from build123d import *

# Parameters (mm, degrees)
F2_DEPTH = 5.08
F3_R     = 16.9333333333
F4_DEPTH = 5.08
F5_DEPTH = 5.08


# Not quite as in the source:
# - a variable given as a bare number and used for a length is read in inches; the dataset says mm whatever the document's units were


with BuildPart() as f2:
    # F1 (on Top) → F2 (new body)
    with BuildSketch(Plane.XY):
        with BuildLine():
            ThreePointArc((100.8237705737, -47.527355603), (134.6904372404, -13.6606889364), (100.8237705737, 20.2059777303))
            Line((100.8237705737, 20.2059777303), (-102.3762294263, 20.2059777303))
            ThreePointArc((-102.3762294263, 20.2059777303), (-136.2428960929, -13.6606889364), (-102.3762294263, -47.527355603))
            Line((-102.3762294263, -47.527355603), (100.8237705737, -47.527355603))
        make_face()
    extrude(amount=F2_DEPTH)

    # F3 (on face) → F4 (join)
    with BuildSketch(Plane(origin=(0, 0, 0), x_dir=(1, 0, 0), z_dir=(0, 0, -1))):
        with Locations((-102.3762294263, 13.6606889364)):
            Circle(F3_R)
    extrude(amount=F4_DEPTH)

    # F3 (on face) → F5 (cut)
    with BuildSketch(Plane(origin=(0, 0, 0), x_dir=(1, 0, 0), z_dir=(0, 0, -1))):
        with Locations((100.8237705737, 13.6606889364)):
            Circle(F3_R)
    extrude(amount=-F5_DEPTH, mode=Mode.SUBTRACT)


solid = f2.part
For this review, take the finished solid that the model builds, in its own axes (mm). A direction names the side the tool comes from. Coordinates: 2 decimals unless noted, no trailing zeros. Loops run counter-clockwise (first coordinate to the right, second up) from the corner with the lowest first, then second, coordinate; pieces in that order, holes last. Notation, with made-up numbers: (62, -5) - (84, -5) arc R25 ccw to (84, 30) - close; hole circle Ø9 at (-4.75, 81.25). An arc over 180 degrees is marked (long way). Use a Markdown table: item, result. Add a question column.
Item 1: We need section D-D (x = -26). Give the boundary of the cut face in (y, z), and give its area (3 significant figures).
Item 2: For line 1 (Z direction, x = 40, y = 2.5); line 2 (Y direction, x = 97, z = 2); line 3 (X direction, y = -18.5, z = 0.5), list the stretches that pass through material, from the lowest coordinate up.
Item 3: Mouldability with a two-part tool opening along X and no side actions: class faces 1 (the face through (-3, -13, 0)), 2 (the face through (87.386, -3.357, 2.504)), 3 (the face through (-136.235, -12.916, 2.504)) as pulls with the +X half, pulls with the -X half, needs draft (parallel to the pull), parting line crosses it, or undercut.
Item 4: We need section B-B (x = 97). Give the boundary of the cut face in (y, z), and give its area (3 significant figures).
Item 5: We need section A-A (y = -3). Give the boundary of the cut face in (x, z), and give its area (3 significant figures).
Item 6: Tool access review of faces 4 (the face through (1, 20.206, 3)), 5 (the face through (-115.814, -3.357, -2.504)): name each direction out of +Z, -Z, +X, -X, +Y, -Y from which nothing blocks a thin tool from reaching the whole face with its end or side.
Item 7: We need section C-C (y = -17). Give the boundary of the cut face in (x, z).
Item 8: Insertion check: pin 1 Ø1 at (y, z) = (-10.5, -3.5) entering from +X. The pin has a flat end and moves straight along its axis. Give the tip position at first contact, or say it passes through.
Results list:
| question | item | result |
|---|---|---|
| 1 | outline | (-47.53, 0) - (20.21, 0) - (20.21, 5.08) - (-47.53, 5.08) - close |
| 1 | area | 344 mm^2 |
| 2 | line 1 | z = 0 to 5.08 |
| 2 | line 2 | y = -47.53 to -30.16, 2.84 to 20.21 |
| 2 | line 3 | x = -135.9 to 84.6, 117.05 to 134.34 |
| 3 | face 1 | needs draft |
| 3 | face 2 | undercut |
| 3 | face 3 | pulls with the -X half |
| 4 | outline | (-47.53, 0) - (-30.16, 0) - (-30.16, 5.08) - (-47.53, 5.08) - close; (2.84, 0) - (20.21, 0) - (20.21, 5.08) - (2.84, 5.08) - close |
| 4 | area | 176 mm^2 |
| 5 | outline | (-134.52, 0) - (-115.53, 0) - (-115.53, -5.08) - (-89.22, -5.08) - (-89.22, 0) - (87.67, 0) - (87.67, 5.08) - (-134.52, 5.08) - close; (113.98, 0) - (132.97, 0) - (132.97, 5.08) - (113.98, 5.08) - close |
| 5 | area | 1,360 mm^2 |
| 6 | face 4 | +Z, -Z, +X, -X, +Y |
| 6 | face 5 | -Z |
| 7 | outline | (-136.08, 0) - (-118.98, 0) - (-118.98, -5.08) - (-85.78, -5.08) - (-85.78, 0) - (84.22, 0) - (84.22, 5.08) - (-136.08, 5.08) - close; (117.42, 0) - (134.53, 0) - (134.53, 5.08) - (117.42, 5.08) - close |
| 8 | pin 1 | stops at x = -85.65 |
